The listing builds one solid part. Answer for the finished solid, in the listing's coordinates (mm). Give positions to 0.01 mm unless a question says otherwise; leave off trailing zeros. Order: outer loops, then holes, each group sorted by start corner. A loop starts at its lowest first (then second) coordinate and runs counter-clockwise, first axis right, second up. Notation, with made-up numbers: M 74.5,2 L 105.5,2 A31 ccw 105.5,28 Z; hole C 66,63 d8. An arc over 180 degrees is marked long. Answer as a JSON object with one key per item and string values. Group by question number.
```python
from build123d import *

# Parameters (mm, degrees)
SKETCH1_W           = 220
SKETCH1_H           = 272
SKETCH1_R           = 2.25
SKETCH1_R_2         = 2.235
SKETCH1_R_3         = 2.24
SKETCH1_R_4         = 2.5
SKETCH1_W_2         = 32
SKETCH1_H_2         = 18
BOSS_EXTRUDE1_DEPTH = 5
CUT_EXTRUDE1_DEPTH  = 175.988571055


with BuildPart() as part:
    # Sketch1 → Boss-Extrude1 (new body)
    with BuildSketch(Plane(origin=(0, 0, 0), x_dir=(1, 0, 0), z_dir=(0, 1, 0))):
        Rectangle(SKETCH1_W, SKETCH1_H)
        with Locations(Location((68, 94, 0), (0, 0, 270))):
            Circle(SKETCH1_R, mode=Mode.SUBTRACT)
        with Locations(Location((76, 104, 0), (0, 0, 270))):
            Circle(SKETCH1_R_2, mode=Mode.SUBTRACT)
        with Locations(Location((76, 84, 0), (0, 0, 270))):
            Circle(SKETCH1_R_3, mode=Mode.SUBTRACT)
        with Locations(Location((-76, 84, 0), (0, 0, 270))):
            Circle(SKETCH1_R, mode=Mode.SUBTRACT)
        with Locations(Location((-68, 94, 0), (0, 0, 270))):
            Circle(SKETCH1_R, mode=Mode.SUBTRACT)
        with Locations(Location((-76, 104, 0), (0, 0, 270))):
            Circle(SKETCH1_R, mode=Mode.SUBTRACT)
        with Locations(Location((-81, 67.5, 0), (0, 0, 270))):
            Circle(SKETCH1_R, mode=Mode.SUBTRACT)
        with Locations(Location((-81, 36.5, 0), (0, 0, 270))):
            Circle(SKETCH1_R, mode=Mode.SUBTRACT)
        with Locations(Location((-59, 67.5, 0), (0, 0, 270))):
            Circle(SKETCH1_R, mode=Mode.SUBTRACT)
        with Locations(Location((-59, 36.5, 0), (0, 0, 270))):
            Circle(SKETCH1_R, mode=Mode.SUBTRACT)
        with Locations(Location((59, 36.5, 0), (0, 0, 270))):
            Circle(SKETCH1_R, mode=Mode.SUBTRACT)
        with Locations(Location((59, 67.5, 0), (0, 0, 270))):
            Circle(SKETCH1_R, mode=Mode.SUBTRACT)
        with Locations(Location((81, 67.5, 0), (0, 0, 270))):
            Circle(SKETCH1_R, mode=Mode.SUBTRACT)
        with Locations(Location((81, 36.5, 0), (0, 0, 270))):
            Circle(SKETCH1_R, mode=Mode.SUBTRACT)
        with Locations(Location((-24.269619723, -13, 0), (0, 0, 270))):
            Circle(SKETCH1_R, mode=Mode.SUBTRACT)
        with Locations(Location((16.730380277, -13, 0), (0, 0, 270))):
            Circle(SKETCH1_R, mode=Mode.SUBTRACT)
        with Locations(Location((-17.315138118, -102.104616257, 0), (0, 0, 270))):
            Circle(SKETCH1_R_4, mode=Mode.SUBTRACT)
        with Locations(Location((17.315138118, -102.104616257, 0), (0, 0, 270))):
            Circle(SKETCH1_R_4, mode=Mode.SUBTRACT)
        with Locations(Location((17.315138118, -73.368855125, 0), (0, 0, 270))):
            Circle(SKETCH1_R_4, mode=Mode.SUBTRACT)
        with Locations(Location((-17.315138118, -73.368855125, 0), (0, 0, 270))):
            Circle(SKETCH1_R_4, mode=Mode.SUBTRACT)
        with Locations(Location((-88.5, 0, 0), (0, 0, 270))):
            Circle(SKETCH1_R_4, mode=Mode.SUBTRACT)
        with Locations(Location((-92.5, 25, 0), (0, 0, 270))):
            Circle(SKETCH1_R_4, mode=Mode.SUBTRACT)
        with Locations(Location((-92.5, -25, 0), (0, 0, 270))):
            Circle(SKETCH1_R_4, mode=Mode.SUBTRACT)
        with Locations((-3.769619723, -13)):
            Rectangle(SKETCH1_W_2, SKETCH1_H_2, mode=Mode.SUBTRACT)
    extrude(amount=BOSS_EXTRUDE1_DEPTH)

    # Sketch3 → Cut-Extrude1 (cut, through all)
    with BuildSketch(Plane(origin=(0, 5, 0), x_dir=(1, 0, 0), z_dir=(0, 1, 0))):
        Polygon((0, 136), (40, 136), (40, -4), (-40, -4), (-40, 136), align=None)
    extrude(amount=-CUT_EXTRUDE1_DEPTH, mode=Mode.SUBTRACT)


solid = part.part
```
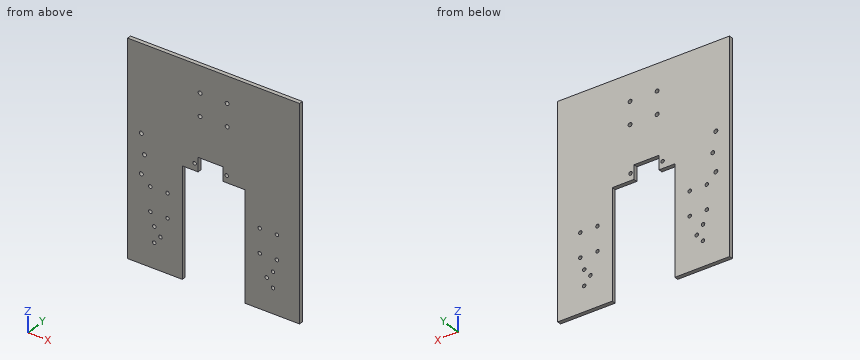
Item 1: Section C-C (y = 3.3) is taken. Count the separate pieces of the cut face and the enclosed holes in it, and give its area (3 significant figures).
Item 2: Flat-ended cylindrical pins translate along their axes: P1, Ø1.5, axis at x = -32.5, y = 2, coming from the -Z side; P2, Ø6, axis at x = -59, z = -67.5, coming from the +Y side; P3, Ø3, axis at x = -17.32, z = 102.1, coming from the -Y side. Find the tip coordinate at first contact, or state that the pin passes through.
Item 3: Section A-A (z = -53.5) is taken. Determine the outline of the cut face in (x, y), and give its area (3 significant figures).
Item 4: Consider probe 1 along Z at (x, y) = (-81.5, 0.3); probe 2 along X at (y, z) = (2.05, 73.5); probe 3 along X at (y, z) = (3.6, -36.5). Determine where each line is inside the solid, lowest interval first. Write a range as from..to.
Item 5: Section B-B (x = 30.5) is taken. Determine the outline of the cut face in (y, z).
Values found:
{
 "1": {"separate pieces": "1", "enclosed holes": "23", "area": "47,700 mm^2"},
 "2": {"P1": "stops at z = 4", "P2": "stops at y = 5", "P3": "passes through"},
 "3": {"outline": "M -110,0 L -40,0 L -40,5 L -110,5 Z; M 40,0 L 110,0 L 110,5 L 40,5 Z", "area": "700 mm^2"},
 "4": {"probe 1": "z = -136..-69.69, -65.31..-38.69, -34.31..136", "probe 2": "x = -110..-19.81, -14.82..14.82, 19.81..110", "probe 3": "x = -110..-83.25, -78.75..-61.25, -56.75..-40, 40..56.75, 61.25..78.75, 83.25..110"},
 "5": {"outline": "M 0,4 L 5,4 L 5,136 L 0,136 Z"}
}
